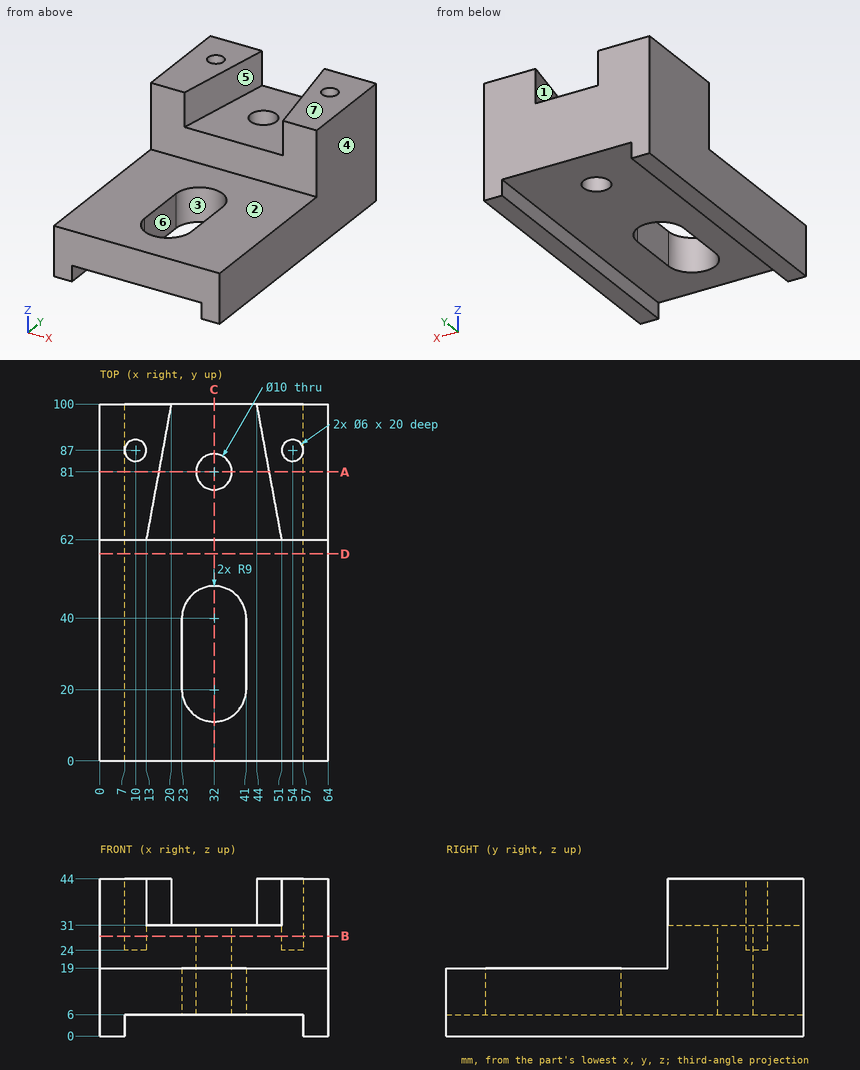
Input: dimensioned drawing with shaded views. Units: mm. Origin: part minimum x, y, z. A direction names the side the tool comes from. Give positions to 0.01 mm unless a question says otherwise; leave off trailing zeros. Order: outer loops, then holes, each group sorted by start corner. A loop starts at its lowest first (then second) coordinate and runs counter-clockwise, first axis right, second up. Notation, with made-up numbers: (25, -1.75) -> (43, -1.75) arc R32 cw to (43, 27.25) -> close; hole circle Ø7 at (72, 87.25). An arc over 180 degrees is marked (long way). Answer as a JSON object with one key per item and string values.
Q1. Section A-A (y = 81). Output: boundary loops of the cut face in (x, z).
Entries:
{"outline": "(0, 0) -> (7, 0) -> (7, 6) -> (27, 6) -> (27, 31) -> (16.5, 31) -> (16.5, 44) -> (0, 44) -> close; (37, 6) -> (57, 6) -> (57, 0) -> (64, 0) -> (64, 44) -> (47.5, 44) -> (47.5, 31) -> (37, 31) -> close"}
Q2. Section B-B (z = 28). Output: boundary loops of the cut face in (x, y), plus the area to 3 significant figures.
Entries:
{"outline": "(0, 62) -> (64, 62) -> (64, 100) -> (0, 100) -> close; hole circle Ø6 at (10, 87); hole circle Ø10 at (32, 81); hole circle Ø6 at (54, 87)", "area": "2,300 mm^2"}
Q3. Section C-C (x = 32). Output: boundary loops of the cut face in (y, z).
Entries:
{"outline": "(0, 6) -> (11, 6) -> (11, 19) -> (0, 19) -> close; (49, 6) -> (76, 6) -> (76, 31) -> (62, 31) -> (62, 19) -> (49, 19) -> close; (86, 6) -> (100, 6) -> (100, 31) -> (86, 31) -> close"}
Q4. Section D-D (y = 58). Output: boundary loops of the cut face in (x, z), plus the area to 3 significant figures.
Entries:
{"outline": "(0, 0) -> (7, 0) -> (7, 6) -> (57, 6) -> (57, 0) -> (64, 0) -> (64, 19) -> (0, 19) -> close", "area": "916 mm^2"}
Q5. Access query for the marked faces 1, 2 and 3. Directions: +Z, -Z, +X, -X, +Y, -Y. A direction counts if a zero-diameter tool reaches every point of the face in a straight line with its end or side. Return the directions, or none.
Entries:
{"face 1": "+Z, -Y", "face 2": "+Z, +X, -X, -Y", "face 3": "+Z, -Z"}
Q6. Material intervals for probe 1 along X at (y, z) = (25.5, 10.5); probe 2 along Y at (x, z) = (10, 29); probe 3 along Z at (x, y) = (60, 10.5), sorted ascending.
Entries:
{"probe 1": "x = 0 to 23, 41 to 64", "probe 2": "y = 62 to 84, 90 to 100", "probe 3": "z = 0 to 19"}
Q7. Draft query along X for the marked faces 4, 5, 6 and 7. Return one class per face: released by +X, released by -X, zero draft, split by the parting line, or undercut.
Entries:
{"face 4": "released by +X", "face 5": "undercut", "face 6": "undercut", "face 7": "zero draft"}
Q8. First-contact query: pin 1 (18.5 mm diameter, centred on x = 17, y = 45.5, fed in from +Z); pin 2 (1.8 mm diameter, centred on x = 53, y = 86.5, fed in from +Z); pin 3 (8 mm diameter, centred on x = 9.5, z = 25, fed in from -Y). Flat tips, straight axial feed; report the tip coordinate or a pass-through.
Entries:
{"pin 1": "stops at z = 19", "pin 2": "stops at z = 24", "pin 3": "stops at y = 62"}
